from build123d import *

# Parameters (mm, degrees)
BOSS_EXTRUDE1_DEPTH     = 12.7
CUT_EXTRUDE1_DEPTH      = 188.996466057
CUT_EXTRUDE1_DEPTH_BACK = 188.996466057
SKETCH3_R               = 3.175


with BuildPart() as part:
    # Sketch1 → Boss-Extrude1 (new body)
    with BuildSketch(Plane.XY):
        Polygon((155.575, -88.9), (-152.4, -88.9), (-152.4, 0), (-152.4, 104.775), (155.575, 104.775), (155.575, 0), align=None)
    extrude(amount=BOSS_EXTRUDE1_DEPTH)

    # Sketch3 → Cut-Extrude1 (cut, two sides: drawn at the far end of the back side and taken through both)
    with BuildSketch(Plane.XY.offset(12.7).offset(-CUT_EXTRUDE1_DEPTH_BACK)):
        with Locations((106.975954286, 70.395873002)):
            Circle(SKETCH3_R)
        with Locations((106.975954286, 42.900373002)):
            Circle(SKETCH3_R)
        with Locations((-59.73361009, 43.51546635)):
            Circle(SKETCH3_R)
        with Locations((-59.73361009, -8.87203365)):
            Circle(SKETCH3_R)
        with Locations((-85.92736009, 17.32171635)):
            Circle(SKETCH3_R)
        with Locations((-114.633914907, -45.510351778)):
            Circle(SKETCH3_R)
        with Locations((8.985545702, 53.468225166)):
            Circle(SKETCH3_R)
        with Locations((41.65587457, 60.657920909)):
            Circle(SKETCH3_R)
        with Locations((60.142975062, 4.412421641)):
            Circle(SKETCH3_R)
        with Locations((50.952707496, -32.969269828)):
            Circle(SKETCH3_R)
        with Locations((23.174346831, -6.319418914)):
            Circle(SKETCH3_R)
        with Locations((-37.672139706, 21.75002)):
            Circle(SKETCH3_R)
        with Locations((89.842754417, 91.683154931)):
            Circle(SKETCH3_R)
        with Locations((116.371246163, 94.499523115)):
            Circle(SKETCH3_R)
    extrude(amount=CUT_EXTRUDE1_DEPTH + CUT_EXTRUDE1_DEPTH_BACK, mode=Mode.SUBTRACT)


solid = part.part
The listing builds one solid part. Answer for the finished solid, in the listing's coordinates (mm). Coordinates: 2 decimals unless noted, no trailing zeros. Write each loop counter-clockwise with the first axis right and the second up, starting at its lowest first coordinate (ties: lowest second). Pieces come first, ordered by that corner, then holes. Notation, with made-up numbers: M -25.75,-13.5 L 25.25,-13.5 A13 cw 25.25,-0.5 Z; hole C 39.25,-32.75 d1. An arc over 180 degrees is marked long. Write each question's results on one line, items separated by ' | '.
Item 1: The part is cut by section A-A on x = 116.5. Determine the outline of the cut face in (y, z) (3 decimals), and give its area (3 significant figures).
Answer below:
outline: M -88.9,0 L 91.327,0 L 91.327,12.7 L -88.9,12.7 Z; M 97.672,0 L 104.775,0 L 104.775,12.7 L 97.672,12.7 Z | area: 2,380 mm2
Item 2: For a pull along X with two mould halves and no side action, classify faces 1 (the face through (4, -88.9, 6)), 2 (the face through (155.575, 7, 6)), 3 (the face through (63.076, 3.196, 6.261)) as released by +X, released by -X, zero draft, split by the parting line, or undercut.
Answer below:
face 1: zero draft | face 2: released by +X | face 3: undercut
Item 3: Consider probe 1 along Y at (x, z) = (-60, 10) (3 decimals); probe 2 along X at (y, z) = (43, 6.25) (3 decimals); probe 3 along X at (y, z) = (17.5, 7.5) (3 decimals). Determine where each line is inside the solid, lowest interval first. Write a range as [from, to].
Answer below:
probe 1: [-88.9, -12.036], [-5.708, 40.352], [46.679, 104.775] | probe 2: [-152.4, -62.866], [-56.601, 103.803], [110.149, 155.575] | probe 3: [-152.4, -89.097], [-82.757, 155.575]
